Build history of the part. All positions in model axes, mm. Face numbers are marked on the shaded views. A direction names the side the tool comes from. Round coordinates to 2 decimals unless told otherwise and drop trailing zeros. Loops run counter-clockwise (first coordinate to the right, second up) from the corner with the lowest first, then second, coordinate; pieces in that order, holes last. Notation, with made-up numbers: (-11.5, -34) - (1.5, -34) arc R29 ccw to (1.5, 4) - close; hole circle Ø10 at (41.5, 44). An arc over 180 degrees is marked (long way). One line per question, with ' | ' between items. Start each with the question number.
from build123d import *

# Parameters (mm, degrees)
SKETCH_1_W             = 108
SKETCH_1_H             = 3.75
EXTRUDE_1_DEPTH        = 10
EXTRUDE_2_DEPTH        = 10
PATTERN_LINEAR_1_COUNT = 25
PATTERN_LINEAR_1_PITCH = 3.142
SKETCH_2_R             = 1.6
CUT_EXTRUDE_1_DEPTH    = 10
CUT_EXTRUDE_2_DEPTH    = 2


with BuildPart() as part:
    # Sketch 1 → Extrude 1 (new body)
    with BuildSketch(Plane(origin=(0, 0, 0), x_dir=(1, 0, 0), z_dir=(0, 1, 0))):
        with Locations((54, 1.875)):
            Rectangle(SKETCH_1_W, SKETCH_1_H)
    extrude(amount=EXTRUDE_1_DEPTH)

    # Sketch 1_5 → Extrude 2 (add)
    with BuildSketch(Plane(origin=(0, 0, 0), x_dir=(1, 0, 0), z_dir=(0, 1, 0))):
        Polygon((105.747407554, 3.75), (108, 3.75), (107.181203777, 5.999624134), (106.566203777, 5.999624134), align=None)
    extrude_2 = extrude(amount=EXTRUDE_2_DEPTH)

    # Pattern Linear 1: Extrude 2 ×25
    with Locations(*[(-i * PATTERN_LINEAR_1_PITCH, 0, 0) for i in range(1, PATTERN_LINEAR_1_COUNT)]):
        add(extrude_2)

    # Sketch 2 → Cut-Extrude 1 (cut)
    with BuildSketch(Plane(origin=(0, 0, -3.75), x_dir=(-1, 0, 0), z_dir=(0, 0, -1))):
        with Locations((-10, 5)):
            Circle(SKETCH_2_R)
        with Locations((-20, 5)):
            Circle(SKETCH_2_R)
    extrude(amount=-CUT_EXTRUDE_1_DEPTH, mode=Mode.SUBTRACT)

    # Sketch 3 → Cut-Extrude 2 (cut)
    with BuildSketch(Plane(origin=(0, 0, -3.75), x_dir=(-1, 0, 0), z_dir=(0, 0, -1))):
        Polygon((-21.58771324, 7.75), (-23.175426481, 5), (-21.58771324, 2.25), (-18.41228676, 2.25), (-16.824573519, 5), (-18.41228676, 7.75), align=None)
        Polygon((-11.58771324, 7.75), (-13.175426481, 5), (-11.58771324, 2.25), (-8.41228676, 2.25), (-6.824573519, 5), (-8.41228676, 7.75), align=None)
    extrude(amount=-CUT_EXTRUDE_2_DEPTH, mode=Mode.SUBTRACT)


solid = part.part
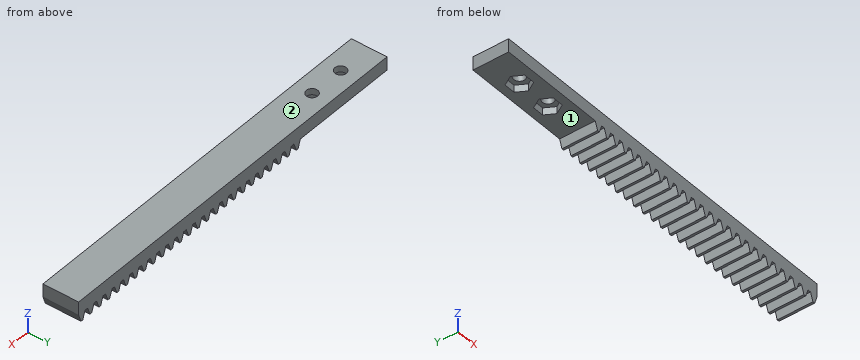
1) Saw through at A-A on x = 20. Write the cut outline in (y, z), and give its area (3 significant figures).
2) Tool access for the marked faces 1 and 2: list every direction of +Z, -Z, +X, -X, +Y, -Y with a clear straight run to the whole face (end or side of a thin tool).
3) Wall check: line 1 (Y direction, x = 20, z = -0.85); line 2 (X direction, y = 5.5, z = -2.85); line 3 (X direction, y = 4, z = -2.35). Give the ranges that are in metal, low to high. Write a range as [from, to].
4) Drop flat-ended pins along their axis: pin 1 (4 mm diameter, centred on x = 10, y = 5, fed in from -Z); pin 2 (0.6 mm diameter, centred on x = 10, z = -2.5, fed in from -Y); pin 3 (0.7 mm diameter, centred on x = 99, y = 5, fed in from -Z). Give the stop position or say it passes through.
Answer key:
1) outline: (0, -3.75) - (2.25, -3.75) - (2.25, -1.75) - (3.4, -1.75) - (3.4, 0) - (0, 0) - close; (6.6, -1.75) - (7.75, -1.75) - (7.75, -3.75) - (10, -3.75) - (10, 0) - (6.6, 0) - close | area: 20.9 mm²
2) face 1: -Z, -X, +Y, -Y | face 2: +Z, +X, -X, +Y, -Y
3) line 1: [0, 3.4], [6.6, 10] | line 2: [0, 7.11], [12.89, 17.11], [22.89, 108] | line 3: [0, 7.4], [12.6, 17.4], [22.6, 108]
4) pin 1: z = -1.75 | pin 2: y = 0 | pin 3: z = -3.75
